from build123d import *

# Parameters (mm, degrees)
SKETCH1_W           = 150
SKETCH1_H           = 100
BOSS_EXTRUDE1_DEPTH = 30
SKETCH3_W           = 20
SKETCH3_H           = 50
REVOLVE1_ANGLE      = 180
CUT_EXTRUDE2_DEPTH  = 198.230829233
CIRPATTERN1_COUNT   = 3
CIRPATTERN1_ANGLE   = 40
CUT_EXTRUDE3_START  = -30
CUT_EXTRUDE3_DEPTH  = 90


with BuildPart() as part:
    # Sketch1 → Boss-Extrude1 (new body)
    with BuildSketch(Plane(origin=(0, 0, 0), x_dir=(1, 0, 0), z_dir=(0, 1, 0))):
        with Locations((75, 50)):
            Rectangle(SKETCH1_W, SKETCH1_H)
    extrude(amount=BOSS_EXTRUDE1_DEPTH)

    # Sketch3 → Revolve1 (revolve)
    with BuildSketch(Plane(origin=(0, 30, 0), x_dir=(1, 0, 0), z_dir=(0, 1, 0))):
        with Locations((140, 75)):
            Rectangle(SKETCH3_W, SKETCH3_H)
        with Locations((10, 75)):
            Rectangle(SKETCH3_W, SKETCH3_H)
    revolve(axis=Axis((150, 30, -50), (1, 0, 0)), revolution_arc=REVOLVE1_ANGLE)

    # Sketch4 → Cut-Extrude2 (cut, through all)
    with BuildSketch(Plane(origin=(150, 0, 0), x_dir=(0, 0, -1), z_dir=(1, 0, 0))):
        Polygon((94.056786042, 54.745020752), (88.321021678, 62.936541195), (73.429921107, 48.847356556), (75.724226853, 45.570748379), align=None)
    cut_extrude2 = extrude(amount=-CUT_EXTRUDE2_DEPTH, mode=Mode.SUBTRACT)

    # CirPattern1: Cut-Extrude2 ×3 about axis
    cirpattern1_axis = Axis((0, 35.163146629, -49.309446005), (1, 0, 0))
    for i in range(1, CIRPATTERN1_COUNT):
        add(cut_extrude2.rotate(cirpattern1_axis, i * CIRPATTERN1_ANGLE / (CIRPATTERN1_COUNT - 1)), mode=Mode.SUBTRACT)

    # Sketch8 → Cut-Extrude3 (cut)
    with BuildSketch(Plane(origin=(150, 0, 0), x_dir=(0, 0, -1), z_dir=(1, 0, 0)).offset(CUT_EXTRUDE3_START)):
        with BuildLine():
            Line((111.193302221, 30), (9.733387686, 30))
            Line((9.733387686, 30), (9.733387686, 6.163594969))
            ThreePointArc((9.733387686, 6.163594969), (54.932592736, 2.173437288), (98.615148428, 14.450400418))
            Line((98.615148428, 14.450400418), (111.193302221, 30))
        make_face()
    extrude(amount=-CUT_EXTRUDE3_DEPTH, mode=Mode.SUBTRACT)


solid = part.part
Read the model definition and answer for the solid it produces. Units are mm, in the model's axes. A direction names the side the tool comes from. Give positions to 0.01 mm unless a question says otherwise; leave off trailing zeros. Write each loop counter-clockwise with the first axis right and the second up, starting at its lowest first coordinate (ties: lowest second). Pieces come first, ordered by that corner, then holes. Notation, with made-up numbers: (6, -33.5) - (12, -33.5) arc R19 cw to (12, -1.5) - close; hole circle Ø11 at (-16, 26). An arc over 180 degrees is marked (long way). Use CSV: the item, a comma, the result in double quotes. Start each with the question number.
Item 1: For faces 5 (the flat face through (71, 30, -9)), 6 (the flat face through (30, 16, -54)), 7 (the cylindrical face through (10.14, 65.01, -85.7)), 8 (the flat face through (10.14, 60.57, -76.81)), determine the directions among +Z, -Z, +X, -X, +Y, -Y from which every point of the face is accessible in a straight line to the end or side of a thin tool.
Item 2: The part is cut by section A-A, the plane y = 18. Give the vertices of the cut face in (x, z).
Item 3: The mould has two halves that part along Z. Classify faces 1 (the flat face through (74, 15, 0)), 2 (the flat face through (10.14, 55.806, -80.784)), 3 (the cylindrical face through (140.1, 74.5, -72.8)), 4 (the flat face through (130, 50, -51)): pulls with the +Z half, pulls with the -Z half, needs draft (parallel to the pull), parting line crosses it, or undercut.
Item 4: The part is cut by section C-C, the plane z = -80. Give the vertices of the cut face in (x, y), and give its area (3 significant figures).
Item 5: The part is cut by section B-B, the plane x = 45.5. Give the vertices of the cut face in (y, z), and give its area (3 significant figures).
Item 6: Consider line 1 (X direction, y = 55.5, z = -16); line 2 (X direction, y = 28, z = -92); line 3 (Y direction, x = 125, z = -40). Determine where each line is inside the solid, lowest interval first.
Item 7: Flat-ended cylindrical pins translate along their axes: P1, Ø7, axis at x = 80, y = 20.5, coming from the -Z side; P2, Ø8, axis at x = 90.5, z = -57, coming from the +Y side. Find the tip coordinate at first contact, or state that the pin passes through.
Item 8: The part is cut by section D-D, the plane y = 43. Give the vertices of the cut face in (x, z).
Taken from the geometry:
1,face 5,"+Z, -Z, +Y"
1,face 6,"+Y"
1,face 7,"-Z, +X, -X, +Y"
1,face 8,"+X, -X"
2,outline,"(0, -100) - (30, -100) - (30, -9.73) - (120, -9.73) - (120, -100) - (150, -100) - (150, 0) - (0, 0) - close"
3,face 1,"pulls with the +Z half"
3,face 2,"undercut"
3,face 3,"pulls with the -Z half"
3,face 4,"needs draft"
4,outline,"(0, 0) - (150, 0) - (150, 47.71) - (130, 47.71) - (130, 30) - (120, 30) - (120, 7.11) - (30, 7.11) - (30, 30) - (20, 30) - (20, 47.71) - (0, 47.71) - close; (0, 55.06) - (20, 55.06) - (20, 63.94) - (0, 63.94) - close; (130, 55.06) - (150, 55.06) - (150, 63.94) - (130, 63.94) - close"
4,area,"3,500 mm2"
5,outline,"(0, -100) - (16.16, -100) - (14.45, -98.62) arc R126.02 cw to (6.16, -9.73) - (30, -9.73) - (30, 0) - (0, 0) - close"
5,area,"740 mm2"
6,line 1,"0 to 20, 130 to 150"
6,line 2,"0 to 30, 120 to 150"
6,line 3,"0 to 30"
7,P1,"z = -9.73"
7,P2,"y = 2.89"
8,outline,"(0, -98.28) - (20, -98.28) - (20, -1.72) - (0, -1.72) - close; (130, -98.28) - (150, -98.28) - (150, -1.72) - (130, -1.72) - close"
